Geometry check sheet. Reference: the model listing, model coordinates, mm. A direction names the side the tool comes from. Give positions to 0.01 mm unless a question says otherwise; leave off trailing zeros. Order: outer loops, then holes, each group sorted by start corner. A loop starts at its lowest first (then second) coordinate and runs counter-clockwise, first axis right, second up.
Autodesk Inventor part; units mm, degrees
ref_plane "Work Plane1" through (0, 87.3125, 0) normal (0, 1, 0) x (1, 0, 0)
ref_plane "YZ Plane" through (0, 0, 0) normal (1, 0, 0) x (0, 1, 0)
ref_plane "XZ Plane" through (0, 0, 0) normal (0, 1, 0) x (-1, 0, 0)
sketch "Sketch1" plane through (0, 0, 0) normal (0, 1, 0) x (-1, 0, 0)
  line L0 (84.9737, 68.5674) -> (-162.6763, 68.5674)
  line L1 (-162.6763, 68.5674) -> (-162.6763, -109.2326)
  line L2 (-162.6763, -109.2326) -> (84.9737, -109.2326)
  line L3 (84.9737, -109.2326) -> (84.9737, 68.5674)
  point P0 (0, 0)
  dimension "d0" = 247.65
  dimension "d1" = 177.8
extrude "Extrusion1" add sketch "Sketch1" along normal blind 4.7625
sketch "Sketch2" plane through (0, 4.7625, 0) normal (0, 1, 0) x (1, 0, 0)
  line L0 (-84.9737, 109.2326) -> (-84.9737, -68.5674)
  line L1 (162.6763, -68.5674) -> (162.6763, 109.2326)
  line L2 (-84.9737, -68.5674) -> (162.6763, -68.5674)
  line L3 (162.6763, -68.5674) -> (162.6763, -63.4874)
  line L4 (162.6763, -63.4874) -> (-84.9737, -63.4874)
  line L5 (-84.9737, -63.4874) -> (-84.9737, -68.5674)
  point P0 (0, 0)
  point P1 (-84.9737, -63.4874)
  dimension "d4" = 5.08
extrude "Extrusion2" add sketch "Sketch2" along normal blind 82.55
sketch "Sketch3" plane through (0, 4.7625, 0) normal (0, 1, 0) x (1, 0, 0)
  line L0 (-84.9737, 109.2326) -> (-84.9737, -68.5674)
  line L1 (162.6763, -68.5674) -> (162.6763, 109.2326)
  line L2 (-84.9737, 109.2326) -> (162.6763, 109.2326)
  line L3 (162.6763, 109.2326) -> (162.6763, 104.1526)
  line L4 (162.6763, 104.1526) -> (-84.9737, 104.1526)
  line L5 (-84.9737, 104.1526) -> (-84.9737, 109.2326)
  point P0 (0, 0)
  point P1 (-84.9737, 104.1526)
  dimension "d7" = 5.08
extrude "Extrusion3" add sketch "Sketch3" along normal blind 82.55
sketch "Sketch4" plane through (0, 4.7625, 0) normal (0, 1, 0) x (1, 0, 0)
  line L0 (-84.9737, -68.5674) -> (162.6763, -68.5674)
  line L1 (162.6763, 109.2326) -> (-84.9737, 109.2326)
  line L2 (-84.9737, -68.5674) -> (-79.8937, -68.5674)
  line L3 (-79.8937, -68.5674) -> (-79.8937, 109.2326)
  line L4 (-79.8937, 109.2326) -> (-84.9737, 109.2326)
  line L5 (-84.9737, 109.2326) -> (-84.9737, -68.5674)
  line L6 (162.6763, -68.5674) -> (157.5963, -68.5674)
  line L7 (157.5963, -68.5674) -> (157.5963, 109.2326)
  line L8 (157.5963, 109.2326) -> (162.6763, 109.2326)
  line L9 (162.6763, 109.2326) -> (162.6763, -68.5674)
  point P0 (0, 0)
  dimension "d10" = 5.08
  dimension "d11" = 5.08
extrude "Extrusion4" add sketch "Sketch4" along normal blind 82.55 contours L5 L1 L3 L0
sketch "Sketch5" plane through (0, 4.7625, 0) normal (0, 1, 0) x (1, 0, 0)
  line L0 (162.6763, 109.2326) -> (-84.9737, 109.2326)
  line L1 (-84.9737, -68.5674) -> (162.6763, -68.5674)
  line L2 (162.6763, 109.2326) -> (157.5963, 109.2326)
  line L3 (157.5963, 109.2326) -> (157.5963, -68.5674)
  line L4 (157.5963, -68.5674) -> (162.6763, -68.5674)
  line L5 (162.6763, -68.5674) -> (162.6763, 109.2326)
  point P0 (0, 0)
  dimension "d14" = 5.08
extrude "Extrusion5" add sketch "Sketch5" along normal blind 82.55
sketch "Sketch6" plane through (-79.8937, 4.7625, -104.1526) normal (0, 0, 1) x (1, 0, 0)
  line L0 (-5.08, -4.7625) -> (-5.08, 82.55)
  line L1 (242.57, -4.7625) -> (242.57, 82.55)
  line L2 (-5.08, 82.55) -> (242.57, 82.55)
  line L3 (242.57, 82.55) -> (242.57, 76.2)
  line L4 (242.57, 76.2) -> (-5.08, 76.2)
  line L5 (-5.08, 76.2) -> (-5.08, 82.55)
  point P0 (79.8937, -4.7625)
  dimension "d17" = 6.35
extrude "Extrusion6" add sketch "Sketch6" along normal blind 167.64
sketch "Sketch7" plane through (0, 0, 0) normal (0, -1, 0) x (1, 0, 0)
  point P0 (0, 0)
ref_plane "Work Plane1" through (0, 87.3125, 0) normal (0, 1, 0) x (1, 0, 0)
sketch "Sketch10" plane through (0, 87.3125, 0) normal (0, 1, 0) x (1, 0, 0)
  line L0 (-39.4156, 64.7377) -> (-51.6456, 64.7377) construction
  spline S0 degree 4 poles (-39.4156, 64.7377) (-51.6456, 64.7377) (-57.2894, 57.2798) (-57.2894, 50.8338) (-49.9984, 47.0841) knots 1 1 1 1 1 2 2 2 2 2
  line L1 (-51.6456, 64.7377) -> (-57.2894, 57.2798) construction
  line L2 (-57.2894, 57.2798) -> (-57.2894, 50.8338) construction
  line L3 (-57.2894, 50.8338) -> (-49.9984, 47.0841) construction
  line L4 (-46.1883, 71.1757) -> (-54.4299, 71.1757) construction
  spline S1 degree 4 poles (-46.1883, 71.1757) (-54.4299, 71.1757) (-64.3781, 58.0298) (-64.3781, 51.5837) (-58.1641, 45.0485) knots 1 1 1 1 1 2 2 2 2 2
  line L5 (-54.4299, 71.1757) -> (-64.3781, 58.0298) construction
  line L6 (-64.3781, 58.0298) -> (-64.3781, 51.5837) construction
  line L7 (-64.3781, 51.5837) -> (-58.1641, 45.0485) construction
  line L8 (-39.4156, 64.7377) -> (27.0232, 64.7377) construction
  spline S2 degree 2 poles (-39.4156, 64.7377) (27.0232, 64.7377) (46.0385, 54.8414) knots 1 1 1 2 2 2
  line L9 (27.0232, 64.7377) -> (46.0385, 54.8414) construction
  spline S3 degree 2 poles (-46.1883, 71.1757) (28.5034, 71.1757) (49.3836, 61.2115) knots 1 1 1 2 2 2
  line L10 (-46.1883, 71.1757) -> (28.5034, 71.1757) construction
  line L11 (28.5034, 71.1757) -> (49.3836, 61.2115) construction
  arc A0 (-58.1641, 45.0485) -> (-49.9984, 47.0841) centre (-54.6585, 48.3817) ccw
  arc A1 (46.0385, 54.8414) -> (49.3836, 61.2115) centre (47.6993, 58.0326) ccw
  line L12 (102.1246, -24.7938) -> (35.8412, -20.2518) construction
  spline S4 degree 2 poles (102.1246, -24.7938) (35.8412, -20.2518) (17.547, -9.0787) knots 1 1 1 2 2 2
  line L13 (35.8412, -20.2518) -> (17.547, -9.0787) construction
  spline S5 degree 2 poles (109.401, -29.8059) (34.884, -24.6997) (14.7339, -13.3314) knots 1 1 1 2 2 2
  line L14 (109.401, -29.8059) -> (34.884, -24.6997) construction
  line L15 (34.884, -24.6997) -> (14.7339, -13.3314) construction
  line L16 (120.9071, -12.1443) -> (113.8896, -7.905) construction
  spline S6 degree 4 poles (102.1246, -24.7938) (114.326, -25.6299) (120.4665, -18.5753) (120.9071, -12.1443) (113.8896, -7.905) knots 1 1 1 1 1 2 2 2 2 2
  line L17 (102.1246, -24.7938) -> (114.326, -25.6299) construction
  line L18 (114.326, -25.6299) -> (120.4665, -18.5753) construction
  line L19 (120.4665, -18.5753) -> (120.9071, -12.1443) construction
  line L20 (127.928, -13.3771) -> (122.1753, -6.4323) construction
  spline S7 degree 4 poles (109.401, -29.8059) (116.796, -30.3126) (127.4874, -19.8081) (127.928, -13.3771) (122.1753, -6.4323) knots 1 1 1 1 1 2 2 2 2 2
  line L21 (109.401, -29.8059) -> (116.796, -30.3126) construction
  line L22 (116.796, -30.3126) -> (127.4874, -19.8081) construction
  line L23 (127.4874, -19.8081) -> (127.928, -13.3771) construction
  arc A2 (122.1753, -6.4323) -> (113.8896, -7.905) centre (118.45, -9.5182) ccw
  arc A3 (17.547, -9.0787) -> (14.7339, -13.3314) centre (16.2173, -11.2559) ccw
  point P0 (0, 0)
  point P1 (0, 194.8532)
extrude "Extrusion9" cut sketch "Sketch10" against normal blind 25.4
properties part number "CigarBox" material "Wood (Maple)"
Item 1: Set-up check for faces 4 (the flat face through (37, 87.312, -22)), 5 (the flat face through (41, 80.962, -22)), 6 (the cylindrical face through (50.847, 84.182, -56.291)): record each of +Z, -Z, +X, -X, +Y, -Y from which the full face is reachable in a straight line by a thin tool's end or side.
Reported:
face 4: +Z, -Z, +X, -X, +Y
face 5: none
face 6: +Y
Item 2: Sectioned sample at B-B (z = 37). Enter the section's corners in (x, y).
Reported:
outline: (-84.97, 0) - (162.68, 0) - (162.68, 87.31) - (-84.97, 87.31) - close; hole (-79.89, 4.76) - (157.6, 4.76) - (157.6, 80.96) - (-79.89, 80.96) - close
Item 3: Draft check along X on faces 1 (the flat face through (162.676, 43, -19)), 2 (the flat face through (37, 43, -109.233)), 3 (the flat face through (-79.894, 42, -19)). Enter one of: released by +X, released by -X, zero draft, split by the parting line, or undercut.
Reported:
face 1: released by +X
face 2: zero draft
face 3: undercut
Item 4: Sectioned sample at A-A (y = 23). Enter the section's corners in (x, z).
Reported:
outline: (-84.97, -109.23) - (162.68, -109.23) - (162.68, 68.57) - (-84.97, 68.57) - close; hole (-79.89, -104.15) - (157.6, -104.15) - (157.6, 63.49) - (-79.89, 63.49) - close
Item 5: Scan lines: L1, parallel to Y at x = 44, z = -1; L2, parallel to Z at x = -16, y = 71; L3, parallel to X at y = 63.5, z = -43. Record each from-to range of solid material in increasing order.
Reported:
L1: y = 0 to 4.76, 80.96 to 87.31
L2: z = -109.23 to -104.15, 63.49 to 68.57
L3: x = -84.97 to -79.89, 157.6 to 162.68
